from build123d import *

# Parameters (mm, degrees)
SKETCH_R        = 7
SKETCH_R_2      = 3
PAD_DEPTH       = 25
SKETCH001_R     = 25
PAD001_DEPTH    = 10
SKETCH002_W     = 35
SKETCH002_H     = 36
POCKET_DEPTH    = 30.001
SKETCH003_R     = 7
POCKET001_DEPTH = 25.001
SKETCH004_R     = 6
POCKET002_DEPTH = 10.001
SKETCH005_W     = 10
SKETCH005_H     = 50
PAD002_DEPTH    = 10
SKETCH006_R     = 10
POCKET003_DEPTH = 10
SKETCH007_W     = 3
SKETCH007_H     = 30
POCKET004_DEPTH = 80.001


with BuildPart() as part:
    # Sketch → Pad (new body, symmetric)
    with BuildSketch(Plane.XZ):
        with BuildLine():
            Line((0, 0), (0, 5))
            Line((0, 5), (6, 5))
            Line((6, 5), (6, 33.000004))
            ThreePointArc((30, 45.012649), (8.286148, 58.41358), (6, 33.000004))
            Line((30, 45.012649), (30, 10))
            Line((30, 10), (55, 10))
            Line((55, 10), (55, 0))
            Line((0, 0), (55, 0))
        make_face()
        with Locations((15.000005, 45)):
            Circle(SKETCH_R, mode=Mode.SUBTRACT)
        with Locations((18, 10)):
            Circle(SKETCH_R_2, mode=Mode.SUBTRACT)
    extrude(amount=PAD_DEPTH, both=True)

    # Sketch001 → Pad001 (new body)
    with BuildSketch(Plane(origin=(0, 0, 10), x_dir=(-1, 0, 0), z_dir=(0, 0, 1))):
        with Locations((-55, 0)):
            Circle(SKETCH001_R)
    extrude(amount=-PAD001_DEPTH)

    # Sketch002 → Pocket (cut, through all)
    with BuildSketch(Plane(origin=(30, 0, 0), x_dir=(0, 0, 1), z_dir=(1, 0, 0))):
        with Locations((42.5, 0)):
            Rectangle(SKETCH002_W, SKETCH002_H)
    extrude(amount=-POCKET_DEPTH, mode=Mode.SUBTRACT)

    # Sketch003 → Pocket001 (cut, through all)
    with BuildSketch(Plane(origin=(0, 0, 25), x_dir=(-1, 0, 0), z_dir=(0, 0, 1))):
        with Locations((-17, 0)):
            Circle(SKETCH003_R)
    extrude(amount=-POCKET001_DEPTH, mode=Mode.SUBTRACT)

    # Sketch004 → Pocket002 (cut, through all)
    with BuildSketch(Plane(origin=(0, 0, 10), x_dir=(-1, 0, 0), z_dir=(0, 0, 1))):
        with Locations((-55, 0)):
            Circle(SKETCH004_R)
    extrude(amount=-POCKET002_DEPTH, mode=Mode.SUBTRACT)

    # Sketch005 → Pad002 (new body)
    with BuildSketch(Plane(origin=(30, 0, 0), x_dir=(0, 0, 1), z_dir=(1, 0, 0))):
        with Locations((15, 0)):
            Rectangle(SKETCH005_W, SKETCH005_H)
    extrude(amount=PAD002_DEPTH)

    # Sketch006 → Pocket003 (cut)
    with BuildSketch(Plane(origin=(40, 0, 0), x_dir=(0, 0, 1), z_dir=(1, 0, 0))):
        with Locations((20, 0)):
            Circle(SKETCH006_R)
    extrude(amount=-POCKET003_DEPTH, mode=Mode.SUBTRACT)

    # Sketch007 → Pocket004 (cut, through all)
    with BuildSketch(Plane(origin=(0, 0, 0), x_dir=(0, 0, -1), z_dir=(-1, 0, 0))):
        with Locations((-1.5, 0)):
            Rectangle(SKETCH007_W, SKETCH007_H)
    extrude(amount=-POCKET004_DEPTH, mode=Mode.SUBTRACT)


solid = part.part
Verification items for the finished model (mm, model axes). A direction names the side the tool comes from. Give positions to 0.01 mm unless a question says otherwise; leave off trailing zeros. Loops run counter-clockwise (first coordinate to the right, second up) from the corner with the lowest first, then second, coordinate; pieces in that order, holes last.
1) Draft check along X on faces 5 (the flat face through (37, -15, 2)), 6 (the flat face through (40, -15, 15)), 7 (the cylindrical face through (10.534, 2.681, 14.154)). Enter one of: pulls with the +X half, pulls with the -X half, needs draft (parallel to the pull), parting line crosses it, or undercut.
2) Sectioned sample at A-A, the plane y = -4.5. Enter the section's corners in (x, z).
3) Sectioned sample at D-D, the plane z = 21.5. Enter the section's corners in (x, y), then the cut area to 3 significant figures.
4) Sectioned sample at C-C, the plane x = 43. Enter the section's corners in (y, z), then the cut area to 3 significant figures.
5) Depth check by flat-ended pin: pin 1 Ø7 at (x, y) = (14, 7.5) entering from +Z; pin 2 Ø14 at (y, z) = (2, 14.5) entering from -X; pin 3 Ø24 at (x, y) = (29, -5.5) entering from -Z; pin 4 Ø5 at (x, y) = (44.5, -1) entering from -Z. Enter the tip coordinate at first touch or a pass-through.
6) Thickness scan on line 1 along X through (y, z) = (-23.25, 45); line 2 along Y through (x, z) = (13, 18.5); line 3 along Y through (x, z) = (26, 51.5). Record the ranges inside material, lowest first.
7) Set-up check for faces 1 (the flat face through (37, 15, 2)), 2 (the flat face through (40, 15, 15)), 3 (the flat face through (24, 4, 25)), 4 (the flat face through (21, -25, 23)): record each of +Z, -Z, +X, -X, +Y, -Y from which the full face is reachable in a straight line by a thin tool's end or side.
8) Sectioned sample at B-B, the plane z = 42. Enter the section's corners in (x, y).
Answers:
1. face 5: needs draft
1. face 6: pulls with the +X half
1. face 7: undercut
2. outline: (0, 3) - (11.64, 3) - (11.64, 25) - (6, 25) - (6, 5) - (0, 5) - close; (22.36, 3) - (51.03, 3) - (51.03, 10) - (40, 10) - (40, 11.07) - (30, 11.07) - (30, 25) - (22.36, 25) - close; (58.97, 3) - (79.59, 3) - (79.59, 10) - (58.97, 10) - close
3. outline: (6, -25) - (30, -25) - (30, 25) - (6, 25) - close; hole circle Ø14 at (17, 0)
3. area: 1,050 mm2
4. outline: (-25, 0) - (-15, 0) - (-15, 3) - (15, 3) - (15, 0) - (25, 0) - (25, 10) - (-25, 10) - close
4. area: 410 mm2
5. pin 1: stops at z = 25
5. pin 2: stops at x = 6
5. pin 3: stops at z = 0
5. pin 4: stops at z = 3
6. line 1: x = 0 to 8, 22 to 30
6. line 2: y = -25 to -5.74, 5.74 to 25
6. line 3: y = -25 to -18, 18 to 25
7. face 1: -Z, +X, -X
7. face 2: +Z, +X, +Y, -Y
7. face 3: +Z, +X, -X
7. face 4: +Z, -Z, +X, -X, -Y
8. outline: (0.3, -25) - (8.68, -25) - (8.68, -18) - (0.3, -18) - close; (0.3, 18) - (8.68, 18) - (8.68, 25) - (0.3, 25) - close; (21.32, -25) - (30, -25) - (30, -18) - (21.32, -18) - close; (21.32, 18) - (30, 18) - (30, 25) - (21.32, 25) - close
